Design review of the part built by this model. Coordinates are the model's own, in mm. A direction names the side the tool comes from. Give positions to 0.01 mm unless a question says otherwise; leave off trailing zeros. Loops run counter-clockwise (first coordinate to the right, second up) from the corner with the lowest first, then second, coordinate; pieces in that order, holes last. Notation, with made-up numbers: M 33.25,56 L 64.25,56 A33 ccw 64.25,92 Z; hole C -34,26 d2. An arc over 180 degrees is marked long. Use a Markdown table: item, result. Add a question column.
(1) Draft analysis for pull direction Y (two halves, no side actions). For faces 1 (the face through (52.5, 8, 5)), 2 (the face through (47.482, -32.871, 3.944)), 3 (the face through (-1, 1, 0)), state which applies: pulls with the +Y half, pulls with the -Y half, needs draft (parallel to the pull), parting line crosses it, or undercut.
(2) Add section C-C, the plane x = 0. Give the boundary of the cut face in (y, z), then the cut area to 4 significant figures.
(3) Insertion check: pin 1 Ø1.6 at (y, z) = (28.5, 3.5) entering from -X; pin 2 Ø14 at (x, y) = (-18, -21) entering from +Z; pin 3 Ø1.5 at (x, y) = (17, -22.5) entering from +Z. Each pin has a flat end and moves straight along its axis. Give the tip position at first contact, or say it passes through.
(4) For faces 4 (the face through (0, 36, 8)), 5 (the face through (40.72, 25.49, 3.49)), list the 3-axis set-ups (+Z, -Z, +X, -X, +Y, -Y) from which the entire face can be reached by the end or side of a thin tool; tool diameter is ignored.
(5) Add section B-B, the plane y = -12.5. Give the boundary of the cut face in (x, z).
(6) Add section D-D, the plane y = 33. Give the boundary of the cut face in (x, z).
(7) Add section A-A, the plane x = -25. Give the boundary of the cut face in (y, z).
(8) For probe 1 along Y at (x, z) = (3, 2.75); probe 2 along Y at (x, z) = (-16, 5.5); probe 3 along X at (y, z) = (19, 3.75), list the stretches that pass through material, from the lowest coordinate up.
```python
from build123d import *

# Parameters (mm, degrees)
F1_DEPTH = 8
F2_T     = -2.5
F4_DEPTH = 2
F6_DEPTH = 5.5


with BuildPart() as f1:
    # F0 (on Top) → F1 (new body)
    with BuildSketch(Plane.XY):
        with BuildLine():
            Line((-30, -40), (30, -40))
            ThreePointArc((30, -40), (47.6776695297, -32.6776695297), (55, -15))
            Line((55, -15), (55, 15))
            ThreePointArc((55, 15), (47.6776695297, 32.6776695297), (30, 40))
            Line((30, 40), (-30, 40))
            ThreePointArc((-30, 40), (-47.6776695297, 32.6776695297), (-55, 15))
            Line((-55, 15), (-55, -15))
            ThreePointArc((-55, -15), (-47.6776695297, -32.6776695297), (-30, -40))
        make_face()
    extrude(amount=F1_DEPTH)

    # F2
    f2_openings = [f1.faces().sort_by_distance(p)[0] for p in [
        (0, 0, 8),
    ]]
    offset(amount=F2_T, openings=f2_openings)

    # F3 (on face) → F4 (join)
    with BuildSketch(Plane.XY.offset(2.5)):
        with BuildLine():
            Line((-45, 15), (-45, 2.5))
            Line((-45, 2.5), (-40, 2.5))
            Line((-40, 2.5), (-40, 15))
            ThreePointArc((-40, 15), (-37.0710678119, 22.0710678119), (-30, 25))
            Line((-30, 25), (-2.5, 25))
            Line((-2.5, 25), (-2.5, 30))
            Line((-2.5, 30), (-30, 30))
            ThreePointArc((-30, 30), (-40.6066017178, 25.6066017178), (-45, 15))
        make_face()
        with BuildLine():
            Line((40, 2.5), (45, 2.5))
            Line((45, 2.5), (45, 15))
            ThreePointArc((45, 15), (40.6066017178, 25.6066017178), (30, 30))
            Line((30, 30), (2.5, 30))
            Line((2.5, 30), (2.5, 25))
            Line((2.5, 25), (30, 25))
            ThreePointArc((30, 25), (37.0710678119, 22.0710678119), (40, 15))
            Line((40, 15), (40, 2.5))
        make_face()
        with BuildLine():
            Line((2.5, -30), (30, -30))
            ThreePointArc((30, -30), (40.6066017178, -25.6066017178), (45, -15))
            Line((45, -15), (45, -2.5))
            Line((45, -2.5), (40, -2.5))
            Line((40, -2.5), (40, -15))
            ThreePointArc((40, -15), (37.0710678119, -22.0710678119), (30, -25))
            Line((30, -25), (2.5, -25))
            Line((2.5, -25), (2.5, -30))
        make_face()
        with BuildLine():
            Line((-30, -30), (-2.5, -30))
            Line((-2.5, -30), (-2.5, -25))
            Line((-2.5, -25), (-30, -25))
            ThreePointArc((-30, -25), (-37.0710678119, -22.0710678119), (-40, -15))
            Line((-40, -15), (-40, -2.5))
            Line((-40, -2.5), (-45, -2.5))
            Line((-45, -2.5), (-45, -15))
            ThreePointArc((-45, -15), (-40.6066017178, -25.6066017178), (-30, -30))
        make_face()
    extrude(amount=F4_DEPTH)

    # F5 (on face) → F6 (join, through all)
    with BuildSketch(Plane.XY.offset(2.5)):
        with BuildLine():
            ThreePointArc((-2, 37.5), (0, 35.5), (2, 37.5))
            Line((2, 37.5), (-2, 37.5))
        make_face()
        with BuildLine():
            Line((52.5, -2), (52.5, 2))
            ThreePointArc((52.5, 2), (50.5, 0), (52.5, -2))
        make_face()
        with BuildLine():
            Line((-2, -37.5), (2, -37.5))
            ThreePointArc((2, -37.5), (0, -35.5), (-2, -37.5))
        make_face()
        with BuildLine():
            ThreePointArc((-50.5, 0), (-51.0857864376, 1.4142135624), (-52.5, 2))
            Line((-52.5, 2), (-52.5, -2))
            ThreePointArc((-52.5, -2), (-51.0857864376, -1.4142135624), (-50.5, 0))
        make_face()
    extrude(amount=F6_DEPTH)


solid = f1.part
```
Established:
| question | item | result |
|---|---|---|
| 1 | face 1 | undercut |
| 1 | face 2 | pulls with the -Y half |
| 1 | face 3 | needs draft |
| 2 | outline | M -40,0 L 40,0 L 40,8 L 35.5,8 L 35.5,2.5 L -35.5,2.5 L -35.5,8 L -40,8 Z |
| 2 | area | 249.5 mm^2 |
| 3 | pin 1 | x = -51.53 |
| 3 | pin 2 | z = 4.5 |
| 3 | pin 3 | z = 2.5 |
| 4 | face 4 | +Z, +X, -X, +Y, -Y |
| 4 | face 5 | +Z |
| 5 | outline | M -55,0 L 55,0 L 55,8 L 52.5,8 L 52.5,2.5 L 45,2.5 L 45,4.5 L 40,4.5 L 40,2.5 L -40,2.5 L -40,4.5 L -45,4.5 L -45,2.5 L -52.5,2.5 L -52.5,8 L -55,8 Z |
| 6 | outline | M -47.35,0 L 47.35,0 L 47.35,8 L 43.5,8 L 43.5,2.5 L -43.5,2.5 L -43.5,8 L -47.35,8 Z |
| 7 | outline | M -40,0 L 40,0 L 40,8 L 37.5,8 L 37.5,2.5 L 30,2.5 L 30,4.5 L 25,4.5 L 25,2.5 L -25,2.5 L -25,4.5 L -30,4.5 L -30,2.5 L -37.5,2.5 L -37.5,8 L -40,8 Z |
| 8 | probe 1 | -40 to -37.5, -30 to -25, 25 to 30, 37.5 to 40 |
| 8 | probe 2 | -40 to -37.5, 37.5 to 40 |
| 8 | probe 3 | -54.68 to -52.14, -44.46 to -39.17, 39.17 to 44.46, 52.14 to 54.68 |
